Here's how the part is built. I have some questions about the finished solid (model axes, mm). A direction names the side the tool comes from. Round coordinates to 2 decimals unless told otherwise and drop trailing zeros. Write each loop counter-clockwise with the first axis right and the second up, starting at its lowest first coordinate (ties: lowest second). Pieces come first, ordered by that corner, then holes. Notation, with made-up numbers: (-11, -17.75) -> (19, -17.75) arc R20 ccw to (19, -0.75) -> close; hole circle Ø3 at (82.25, -22.75). An arc over 180 degrees is marked (long way). Answer in a Markdown table with one row per item.
from build123d import *

# Parameters (mm, degrees)
ESQUISSE1_W             = 20
ESQUISSE1_H             = 20
ESQUISSE1_R             = 5
ESQUISSE1_H_2           = 30
BOSS_EXTRU_1_DEPTH      = 15
ESQUISSE2_W             = 20
ESQUISSE2_H             = 50
ESQUISSE2_R             = 5
BOSS_EXTRU_2_DEPTH      = 35
ESQUISSE3_R             = 2.5
ENL_V_MAT_EXTRU_1_DEPTH = 30
ESQUISSE4_W             = 50
ESQUISSE4_H             = 20
ENL_V_MAT_EXTRU_2_DEPTH = 10


with BuildPart() as part:
    # Esquisse1 → Boss.-Extru.1 (new body)
    with BuildSketch(Plane.XY):
        Rectangle(ESQUISSE1_W, ESQUISSE1_H)
        Circle(ESQUISSE1_R, mode=Mode.SUBTRACT)
        with Locations((0, -25)):
            Rectangle(ESQUISSE1_W, ESQUISSE1_H_2)
    extrude(amount=BOSS_EXTRU_1_DEPTH)

    # Esquisse2 → Boss.-Extru.2 (add)
    with BuildSketch(Plane.XY.offset(15)):
        with Locations((0, -15)):
            Rectangle(ESQUISSE2_W, ESQUISSE2_H)
        Circle(ESQUISSE2_R, mode=Mode.SUBTRACT)
    extrude(amount=BOSS_EXTRU_2_DEPTH)

    # Esquisse3 → Enlèv. mat.-Extru.1 (cut)
    with BuildSketch(Plane(origin=(10, 0, 0), x_dir=(0, 0, -1), z_dir=(1, 0, 0))):
        with Locations((-42, -30)):
            Circle(ESQUISSE3_R)
        with Locations((-8, -30)):
            Circle(ESQUISSE3_R)
    extrude(amount=-ENL_V_MAT_EXTRU_1_DEPTH, mode=Mode.SUBTRACT)

    # Esquisse4 → Enlèv. mat.-Extru.2 (cut)
    with BuildSketch(Plane(origin=(10, 0, 0), x_dir=(0, 0, -1), z_dir=(1, 0, 0))):
        with Locations((-25, -30)):
            Rectangle(ESQUISSE4_W, ESQUISSE4_H)
    extrude(amount=-ENL_V_MAT_EXTRU_2_DEPTH, mode=Mode.SUBTRACT)


solid = part.part
1) Which directions (+Z, -Z, +X, -X, +Y, -Y) give clear straight access to the entire face, cutting with the end or side of a thin tool? Please do faces 1 (the face through (5, -20, 25)), 2 (the face through (0, 10, 25)).
Response:
| item | result |
|---|---|
| face 1 | +Z, -Z, +X, -Y |
| face 2 | +Z, -Z, +X, -X, +Y |
2) I want a section at A-A, the plane z = 42. List the corners of the cut face in (x, y) for me, and give its area (3 significant figures).
Response:
| item | result |
|---|---|
| outline | (-10, -40) -> (0, -40) -> (0, -32.5) -> (-10, -32.5) -> close; (-10, -27.5) -> (0, -27.5) -> (0, -20) -> (10, -20) -> (10, 10) -> (-10, 10) -> close; hole circle Ø10 at (0, 0) |
| area | 671 mm^2 |
3) I want a section at C-C, the plane y = 0. List the corners of the cut face in (x, z) for me.
Response:
| item | result |
|---|---|
| outline | (-10, 0) -> (-5, 0) -> (-5, 50) -> (-10, 50) -> close; (5, 0) -> (10, 0) -> (10, 50) -> (5, 50) -> close |
4) I want a section at B-B, the plane x = -4. List the corners of the cut face in (y, z) for me.
Response:
| item | result |
|---|---|
| outline | (-40, 0) -> (-3, 0) -> (-3, 50) -> (-40, 50) -> close; (3, 0) -> (10, 0) -> (10, 50) -> (3, 50) -> close; hole circle Ø5 at (-30, 8); hole circle Ø5 at (-30, 42) |
5) For pin 1 (4.5 mm diameter, centred on y = -30, z = 42, fed in from -X); pin 2 (4 mm diameter, centred on y = -22.5, z = 27, fed in from +X); pin 3 (5 mm diameter, centred on x = 7.5, z = 18.5, fed in from -Y), each with a flat end and sliding along its axis, tell me the tip position at first contact or that it passes through.
Response:
| item | result |
|---|---|
| pin 1 | passes through |
| pin 2 | stops at x = 0 |
| pin 3 | stops at y = -20 |
6) I want a section at D-D, the plane z = 33.5. List the corners of the cut face in (x, y) for me, and give its area (3 significant figures).
Response:
| item | result |
|---|---|
| outline | (-10, -40) -> (0, -40) -> (0, -20) -> (10, -20) -> (10, 10) -> (-10, 10) -> close; hole circle Ø10 at (0, 0) |
| area | 721 mm^2 |
7) I need wall thicknesses on line 1 (Y direction, x = -1.75, z = 8); line 2 (Y direction, x = -4, z = 8); line 3 (X direction, y = -29, z = 13). Which ranges of each line are inside material? Lowest first, please. Write a range as [from, to].
Response:
| item | result |
|---|---|
| line 1 | y = [-40, -32.5], [-27.5, -4.68], [4.68, 10] |
| line 2 | y = [-40, -32.5], [-27.5, -3], [3, 10] |
| line 3 | x = [-10, 0] |
8) We'd pull the mould along Y, two halves only. Please class faces 3 (the face through (-5, -40, 25)), 4 (the face through (-4.93, -27.89, 40.66)), 5 (the face through (0, -30, 25)): +Y half, -Y half, draft (parallel to the pull), parting line (faces both ways), or undercut.
Response:
| item | result |
|---|---|
| face 3 | -Y half |
| face 4 | undercut |
| face 5 | draft |
